```python
from build123d import *

# Parameters (mm, degrees)
F1_R     = 31.75
F2_DEPTH = 7.0555555556
F5_R     = 3.5277777778
F6_DEPTH = 14.1111111111


# Not quite as in the source:
# - a variable given as a bare number and used for a length is read in inches; the dataset says mm whatever the document's units were


with BuildPart() as f2:
    # F1 (on Front) → F2 (new body, symmetric)
    with BuildSketch(Plane.XZ):
        Circle(F1_R)
    extrude(amount=F2_DEPTH, both=True)

    # F3 (on Right) → F4 (revolve, cut)
    with BuildSketch(Plane.YZ):
        with BuildLine():
            Line((3.81, 31.75), (-3.81, 31.75))
            ThreePointArc((-3.81, 31.75), (0, 27.94), (3.81, 31.75))
        make_face()
    revolve(axis=Axis((0, -7.0555555556, 0), (0, -1, 0)), mode=Mode.SUBTRACT)

    # F5 (on face) → F6 (cut, through all)
    with BuildSketch(Plane(origin=(0, 7.0555555556, 0), x_dir=(-1, 0, 0), z_dir=(0, 1, 0))):
        Circle(F5_R)
    extrude(amount=-F6_DEPTH, mode=Mode.SUBTRACT)


solid = f2.part
```
Geometry: final body of the model. Coordinates: model frame, mm. Coordinates: 2 decimals unless noted, no trailing zeros. Loops run counter-clockwise (first coordinate to the right, second up) from the corner with the lowest first, then second, coordinate; pieces in that order, holes last. Notation, with made-up numbers: (13.25, -35.5) -> (42.25, -35.5) arc R27 cw to (42.25, -13.5) -> close; hole circle Ø5 at (61, -33.75). An arc over 180 degrees is marked (long way). Use a Markdown table: item, result. Add a question column.
(1) Section query C-C, the plane y = -0.25. Return loops of the section in (x, z).
(2) Pin query (flat end, axial travel): pin 1 Ø6 at (x, y) = (17, 4.5) entering from -Z; pin 2 Ø3 at (y, z) = (-4.5, 10.5) entering from +X; pin 3 Ø1 at (x, z) = (-21, -25) entering from -Y; pin 4 Ø1.5 at (y, z) = (-5, 22.5) entering from -X. Return the tip coordinate at first contact, or that it passes through.
(3) Section query B-B, the plane z = 0. Return loops of the section in (x, y).
(4) Mould query, pull axis Z, two halves, no side actions, for faces 1 (the cylindrical face through (0.459, 0.099, 3.498)), 2 (the flat face through (7, -7.056, 0)), 3 (the cylindrical face through (30.284, 5.41, 9.537)). Classes: pulls with the +Z half, pulls with the -Z half, needs draft (parallel to the pull), parting line crosses it, or undercut.
(5) Section query D-D, the plane y = 3. Return loops of the section in (x, z), plus the area to 3 significant figures.
(6) Line query: line 1 along Y through (x, z) = (11, -27); line 2 along Z through (x, y) = (0, 2.75); line 3 along Z through (x, y) = (0, 3.25). Output: solid intervals per line, ascending.
(7) Section query A-A, the plane x = 0. Return loops of the section in (y, z), plus the area to 3 significant figures.
Answer:
| question | item | result |
|---|---|---|
| 1 | outline | circle Ø55.9 at (0, 0); hole circle Ø7.06 at (0, 0) |
| 2 | pin 1 | stops at z = -28.5 |
| 2 | pin 2 | stops at x = 30.45 |
| 2 | pin 3 | passes through |
| 2 | pin 4 | stops at x = -23.13 |
| 3 | outline | (-31.75, -7.06) -> (-3.53, -7.06) -> (-3.53, 7.06) -> (-31.75, 7.06) -> (-31.75, 3.81) arc R3.81 cw to (-31.75, -3.81) -> close; (3.53, -7.06) -> (31.75, -7.06) -> (31.75, -3.81) arc R3.81 cw to (31.75, 3.81) -> (31.75, 7.06) -> (3.53, 7.06) -> close |
| 4 | face 1 | undercut |
| 4 | face 2 | needs draft |
| 4 | face 3 | parting line crosses it |
| 5 | outline | circle Ø58.8 at (0, 0); hole circle Ø7.06 at (0, 0) |
| 5 | area | 2,680 mm^2 |
| 6 | line 1 | y = -7.06 to -2.79, 2.79 to 7.06 |
| 6 | line 2 | z = -29.11 to -3.53, 3.53 to 29.11 |
| 6 | line 3 | z = -29.76 to -3.53, 3.53 to 29.76 |
| 7 | outline | (-7.06, -31.75) -> (-3.81, -31.75) arc R3.81 cw to (3.81, -31.75) -> (7.06, -31.75) -> (7.06, -3.53) -> (-7.06, -3.53) -> close; (-7.06, 3.53) -> (7.06, 3.53) -> (7.06, 31.75) -> (3.81, 31.75) arc R3.81 cw to (-3.81, 31.75) -> (-7.06, 31.75) -> close |
| 7 | area | 751 mm^2 |
